Design review of the part built by this model. Coordinates are the model's own, in mm. Give positions to 0.01 mm unless a question says otherwise; leave off trailing zeros. Order: outer loops, then holes, each group sorted by start corner. A loop starts at its lowest first (then second) coordinate and runs counter-clockwise, first axis right, second up.
```python
from build123d import *

# Parameters (mm, degrees)
SKETCH1_W               = 10
SKETCH1_H               = 10
BOSS_EXTRUDE1_DEPTH     = 154
CUT_EXTRUDE1_DEPTH      = 155.405310789
CUT_EXTRUDE1_DEPTH_BACK = 155.405310789
SKETCH2_R               = 4


with BuildPart() as part:
    # Sketch1 → Boss-Extrude1 (new body)
    with BuildSketch(Plane(origin=(0, 0, 0), x_dir=(1, 0, 0), z_dir=(0, 1, 0))):
        Rectangle(SKETCH1_W, SKETCH1_H)
    extrude(amount=BOSS_EXTRUDE1_DEPTH)

    # Sketch2 → Cut-Extrude1 (cut, two sides: drawn at the far end of the back side and taken through both)
    with BuildSketch(Plane(origin=(5, 0, 0), x_dir=(0, 0, -1), z_dir=(1, 0, 0)).offset(-CUT_EXTRUDE1_DEPTH_BACK)):
        with Locations((0, 77)):
            Circle(SKETCH2_R)
    extrude(amount=CUT_EXTRUDE1_DEPTH + CUT_EXTRUDE1_DEPTH_BACK, mode=Mode.SUBTRACT)


solid = part.part
```
1. Take a section at C-C (x = 3.5). State the section outline as (y, z) points.
Recorded:
outline: (0, -5) - (154, -5) - (154, 5) - (0, 5) - close; hole circle Ø8 at (77, 0)
2. Take a section at B-B (y = 77). State the section outline as (x, z) points, then the cut area to 3 significant figures.
Recorded:
outline: (-5, -5) - (5, -5) - (5, -4) - (-5, -4) - close; (-5, 4) - (5, 4) - (5, 5) - (-5, 5) - close
area: 20.0 mm2
3. Draft analysis for pull direction Z (two halves, no side actions). For faces 1 (the face through (-0.07, 73.095, 0.867)), 2 (the face through (0, 76, -5)), 3 (the face through (5, 75.9, -4.4)), state which applies: pulls with the +Z half, pulls with the -Z half, needs draft (parallel to the pull), parting line crosses it, or undercut.
Recorded:
face 1: undercut
face 2: pulls with the -Z half
face 3: needs draft
4. For line 1 along Y through (x, z) = (-2.5, 0); line 2 along Z through (x, y) = (-1.25, 77); line 3 along Y through (x, z) = (0, -1), list the stretches that pass through material, from the lowest coordinate up.
Recorded:
line 1: y = 0 to 73, 81 to 154
line 2: z = -5 to -4, 4 to 5
line 3: y = 0 to 73.13, 80.87 to 154
5. Take a section at A-A (z = 0). State the section outline as (x, y) points.
Recorded:
outline: (-5, 0) - (5, 0) - (5, 73) - (-5, 73) - close; (-5, 81) - (5, 81) - (5, 154) - (-5, 154) - close
